Geometry: final body of the model. Coordinates: model frame, mm. A direction names the side the tool comes from. Round coordinates to 2 decimals unless told otherwise and drop trailing zeros. Order: outer loops, then holes, each group sorted by start corner. A loop starts at its lowest first (then second) coordinate and runs counter-clockwise, first axis right, second up. Notation, with made-up numbers: (53.5, -3.5) -> (91.5, -3.5) arc R25 cw to (91.5, 23.5) -> close; hole circle Ø9 at (65, 54). An arc over 180 degrees is marked (long way). Put each result on its own line as item: value.
```python
from build123d import *

# Parameters (mm, degrees)
F0_W            = 241.3
F0_H            = 22.352
F1_DEPTH        = 127
F2_R            = 15.748
F3_W            = 127
F3_H            = 168.402
F4_DEPTH        = 57.15
F5_R            = 15.748
F7_D            = 6.35
F7_CBORE_D      = 19.05
F7_CBORE_DEPTH  = 6.35
F9_D            = 6.35
F9_CSINK_D      = 21.59
F9_CSINK_ANGLE  = 82
F10_D           = 6.35
F10_CSINK_D     = 21.59
F10_CSINK_ANGLE = 90
F11_D           = 6.35
F11_CBORE_D     = 19.05
F11_CBORE_DEPTH = 6.35


with BuildPart() as f1:
    # F0 (on Right) → F1 (new body)
    with BuildSketch(Plane.YZ):
        with Locations((120.65, 11.176)):
            Rectangle(F0_W, F0_H)
    extrude(amount=-F1_DEPTH)

    # F2
    f2_edges = [f1.edges().sort_by_distance(p)[0] for p in [
        (0, 0, 11.176),
        (-127, 0, 11.176),
    ]]
    fillet(f2_edges, radius=F2_R)

    # F3 (on face) → F4 (join)
    with BuildSketch(Plane.XY.offset(22.352)):
        with Locations((-63.5, 157.099)):
            Rectangle(F3_W, F3_H)
    extrude(amount=F4_DEPTH)

    # F5
    f5_edges = [f1.edges().sort_by_distance(p)[0] for p in [
        (0, 72.898, 50.927),
        (-127, 72.898, 50.927),
        (0, 241.3, 39.751),
        (-127, 241.3, 39.751),
    ]]
    fillet(f5_edges, radius=F5_R)

    # F7 (through all)
    with Locations(Plane.XY.offset(22.352)):
        with Locations((-101.6, 35.052)):
            CounterBoreHole(F7_D / 2, F7_CBORE_D / 2, F7_CBORE_DEPTH)

    # F9 (through all)
    with Locations(Plane.XY.offset(79.502)):
        with Locations((-95.25, 136.652)):
            CounterSinkHole(F9_D / 2, F9_CSINK_D / 2, counter_sink_angle=F9_CSINK_ANGLE)

    # F10 (through all)
    with Locations(Plane.XY.offset(79.502)):
        with Locations((-35.052, 98.552)):
            CounterSinkHole(F10_D / 2, F10_CSINK_D / 2, counter_sink_angle=F10_CSINK_ANGLE)

    # F11 (through all)
    with Locations(Plane.XY.offset(79.502)):
        with Locations((-35.052, 184.15)):
            CounterBoreHole(F11_D / 2, F11_CBORE_D / 2, F11_CBORE_DEPTH)


solid = f1.part
```
1. Cut plane A-A on y = 184.15. Return loops of the section in (x, z).
Ans:
outline: (-127, 0) -> (-38.23, 0) -> (-38.23, 73.15) -> (-44.58, 73.15) -> (-44.58, 79.5) -> (-127, 79.5) -> close; (-31.88, 0) -> (0, 0) -> (0, 79.5) -> (-25.53, 79.5) -> (-25.53, 73.15) -> (-31.88, 73.15) -> close
2. Cut plane D-D on x = -95.25. Return loops of the section in (y, z).
Ans:
outline: (0, 0) -> (133.48, 0) -> (133.48, 70.74) -> (125.86, 79.5) -> (72.9, 79.5) -> (72.9, 22.35) -> (42.15, 22.35) -> (42.15, 16) -> (27.95, 16) -> (27.95, 22.35) -> (0, 22.35) -> close; (139.83, 0) -> (241.3, 0) -> (241.3, 79.5) -> (147.45, 79.5) -> (139.83, 70.74) -> close
3. Contact query for flat-ended pins moving along their axis: P1, Ø5.5, axis at x = -95.25, y = 136.652, coming from the +Z side; P2, Ø17, axis at x = -101.6, y = 35.052, coming from the +Z side; P3, Ø10, axis at x = -102, z = 41.5, coming from the -Y side; P4, Ø1.5, axis at x = -89, y = 141.5, coming from the +Z side. Output: stop coordinate, or through.
Ans:
P1: through
P2: z = 16
P3: y = 72.9
P4: z = 77.05
4. Cut plane B-B on x = -55.5. Return loops of the section in (y, z).
Ans:
outline: (0, 0) -> (241.3, 0) -> (241.3, 79.5) -> (72.9, 79.5) -> (72.9, 22.35) -> (0, 22.35) -> close
5. Material intervals for probe 1 along Y at (x, z) = (-37, 8.5); probe 2 along X at (y, z) = (184, 77); probe 3 along Y at (x, z) = (-73, 55), sorted ascending.
Ans:
probe 1: 0 to 96.04, 101.06 to 181.64, 186.66 to 241.3
probe 2: -127 to -44.58, -25.53 to 0
probe 3: 72.9 to 241.3
6. Set-up query: faces 4 (the face through (-127, 142, 39)), 5 (the face through (-64, 72.898, 51)), 6 (the face through (-37.117, 174.852, 76.371)). Return all of +Z, -Z, +X, -X, +Y, -Y with unobstructed straight access to the full face (end or side cutting, diameter ignored); none if empty.
Ans:
face 4: +Z, -Z, -X, +Y, -Y
face 5: +Z, +X, -X, -Y
face 6: +Z
7. Draft query along Y for faces 1 (the face through (-102, 31, 16.002)), 2 (the face through (-122.509, 77.634, 51.327)), 3 (the face through (-63, 119, 0)). Return one class per face: +Y half, -Y half, draft (parallel to the pull), parting line (faces both ways), or undercut.
Ans:
face 1: undercut
face 2: -Y half
face 3: draft
8. Cut plane C-C on z = 31.5. Return loops of the section in (x, y) (3 decimals).
Ans:
outline: (-127, 88.646) arc R15.748 ccw to (-111.252, 72.898) -> (-15.748, 72.898) arc R15.748 ccw to (0, 88.646) -> (0, 225.552) arc R15.748 ccw to (-15.748, 241.3) -> (-111.252, 241.3) arc R15.748 ccw to (-127, 225.552) -> close; hole circle Ø6.35 at (-95.25, 136.652); hole circle Ø6.35 at (-35.052, 98.552); hole circle Ø6.35 at (-35.052, 184.15)
